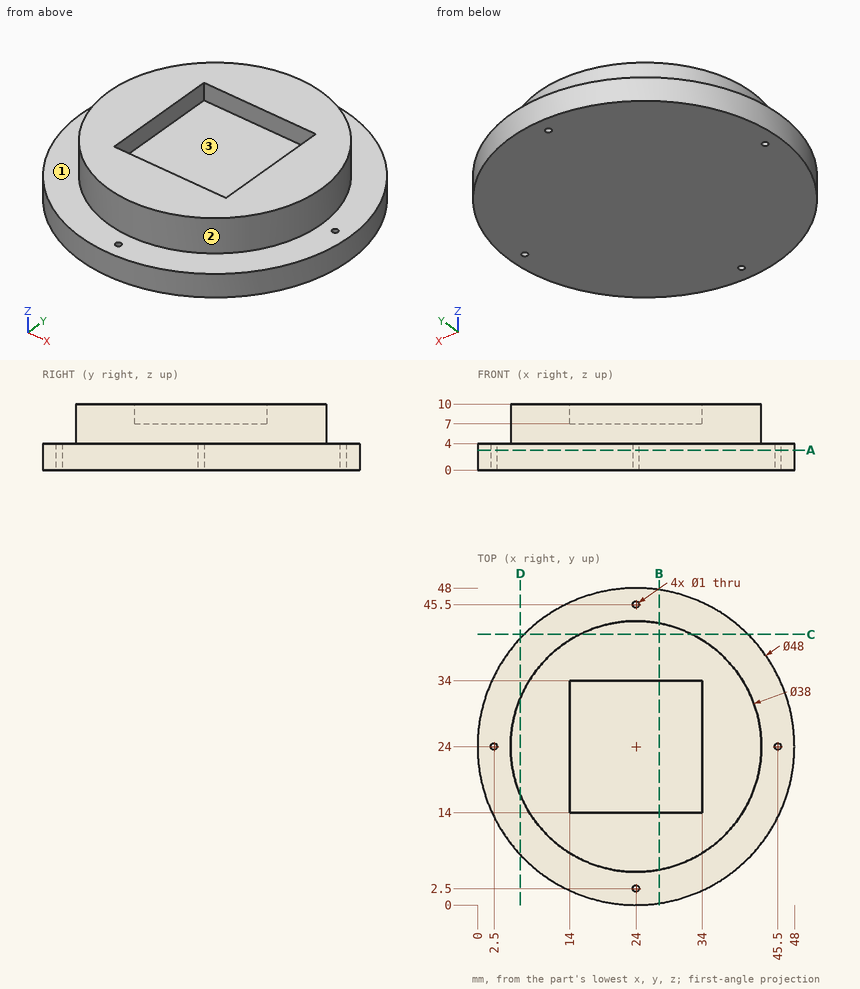
Here's the drawing with two shaded views (mm, measured from the low corner). I have some questions. Coordinates: 2 decimals unless noted, no trailing zeros. Order: outer loops, then holes, each group sorted by start corner. A loop starts at its lowest first (then second) coordinate and runs counter-clockwise, first axis right, second up.
Q1. Suppose I cut it at A-A on z = 3. Please give me the cut outline in (x, y), and give its area (3 significant figures).
Q2. Suppose I cut it at D-D on x = 6.5. Please give me the cut outline in (y, z), and give its area (3 significant figures).
Q3. Suppose I cut it at B-B on x = 27.5. Please give me the cut outline in (y, z).
Q4. Suppose I cut it at C-C on y = 41. Please give me the cut outline in (x, z), and give its area (3 significant figures).
Q5. Please list where these lines run through material, in increasing order: L1, parallel to Y at x = 24, z = 3.1; L2, parallel to X at y = 2.5, z = 1.5.
Q6. Will these pins go through, and if not, where does the flat tip stop? pin 1 (1.5 mm diameter, centred on x = 31.5, z = 7, fed in from -Y); pin 2 (2.5 mm diameter, centred on x = 25, z = 8, fed in from +Y); pin 3 (3 mm diameter, centred on x = 28.5, z = 7, fed in from -Y); pin 4 (8 mm diameter, centred on x = 38.5, y = 19, fed in from -Z).
Q7. Thinking about a two-plate mould opening in Y: for the marked faces 1, 2 and 3, which applies, released by +Y, released by -Y, zero draft, split by the parting line, or undercut?
Answer:
1. outline: circle Ø48 at (24, 24); hole circle Ø1 at (2.5, 24); hole circle Ø1 at (24, 2.5); hole circle Ø1 at (24, 45.5); hole circle Ø1 at (45.5, 24)
1. area: 1,810 mm2
2. outline: (7.58, 0) - (40.42, 0) - (40.42, 4) - (31.4, 4) - (31.4, 10) - (16.6, 10) - (16.6, 4) - (7.58, 4) - close
2. area: 220 mm2
3. outline: (0.26, 0) - (47.74, 0) - (47.74, 4) - (42.67, 4) - (42.67, 10) - (34, 10) - (34, 7) - (14, 7) - (14, 10) - (5.33, 10) - (5.33, 4) - (0.26, 4) - close
4. outline: (7.06, 0) - (40.94, 0) - (40.94, 4) - (32.49, 4) - (32.49, 10) - (15.51, 10) - (15.51, 4) - (7.06, 4) - close
4. area: 237 mm2
5. L1: y = 0 to 2, 3 to 45, 46 to 48
5. L2: x = 13.33 to 23.5, 24.5 to 34.67
6. pin 1: stops at y = 6.24
6. pin 2: stops at y = 43
6. pin 3: stops at y = 5.24
6. pin 4: stops at z = 0
7. face 1: zero draft
7. face 2: split by the parting line
7. face 3: undercut
